Here's how the part is built. I have some questions about the finished solid (model axes, mm). A direction names the side the tool comes from. Coordinates: 2 decimals unless noted, no trailing zeros. Loops run counter-clockwise (first coordinate to the right, second up) from the corner with the lowest first, then second, coordinate; pieces in that order, holes last. Notation, with made-up numbers: (48, 23.25) -> (62, 23.25) arc R19 cw to (62, 31.25) -> close; hole circle Ø8 at (48.25, 10.5). An arc over 180 degrees is marked (long way). Answer as a JSON object with one key per item and string values. Group by question number.
Q1. I'm going to push flat-ended pins straight in: pin 1 (12 mm diameter, centred on x = 52, z = -16.5, fed in from +Y); pin 2 (2.5 mm diameter, centred on x = 1.5, z = -13.5, fed in from +Y); pin 3 (6.5 mm diameter, centred on x = 62.55, z = -35.8, fed in from +Y); pin 4 (3 mm diameter, centred on x = 62.55, z = -15, fed in from -Y). Where does each tip first touch, or does it pass through?
Q2. On a 3-axis mill with a long thin cutter (end or side, diameter ignored), from which of +Z, -Z, +X, -X, +Y, -Y can I reach the whole of each face in a straight line? I mean faces 1 (the flat face through (44, 6.35, -25)), 2 (the cylindrical face through (3.22, 29.41, -14.06)), 3 (the flat face through (3, 71, -15.175)). Say none if no direction works.
Q3. I want a section at D-D on x = 45. Write out the boundary of the cut face in (y, z).
Q4. I want a section at B-B on x = 26.35. Write out the boundary of the cut face in (y, z), then the cut area to 3 significant figures.
Q5. I need wall thicknesses on line 1 (X direction, y = 1.2, z = -15); line 2 (Z direction, x = 62.55, y = 1.2); line 3 (Y direction, x = 2.75, z = -25.4). Which ranges of each line are inside material? Lowest first, please.
Q6. Thinking about a two-plate mould opening in Z: for faces 4 (the flat face through (0, 47, -14)), 5 (the flat face through (23, 4, -50.8)), 6 (the flat face through (3, 71, -12)), 7 (the flat face through (23, 4, 0)), which applies, released by +Z, released by -Z, zero draft, split by the parting line, or undercut?
Q7. I want a section at C-C on z = -25.4. Write out the boundary of the cut face in (x, y), then the cut area to 3 significant figures.
Q8. I want a section at A-A on y = 38.1. Write out the boundary of the cut face in (x, z).
```python
from build123d import *

# Parameters (mm, degrees)
SKETCH1_W                                          = 50.8
SKETCH1_H                                          = 76.2
BOSS_EXTRUDE1_DEPTH                                = 6.35
SKETCH2_W                                          = 50.8
SKETCH2_H                                          = 6.35
BOSS_EXTRUDE2_DEPTH                                = 76.2
SKETCH3_R                                          = 14.2875
CUT_EXTRUDE1_DEPTH                                 = 7.35
CSK_FOR_10_FLAT_HEAD_SOCKET_CAP_SCREW1_D           = 5.1054
CSK_FOR_10_FLAT_HEAD_SOCKET_CAP_SCREW1_CSINK_D     = 10.4394
CSK_FOR_10_FLAT_HEAD_SOCKET_CAP_SCREW1_CSINK_ANGLE = 82
SKETCH12_W                                         = 3.175
SKETCH12_H                                         = 10.4
CUT_EXTRUDE2_DEPTH                                 = 7.35


with BuildPart() as part:
    # Sketch1 → Boss-Extrude1 (new body)
    with BuildSketch(Plane(origin=(0, 0, 0), x_dir=(0, 0, -1), z_dir=(1, 0, 0))):
        with Locations((25.4, 38.1)):
            Rectangle(SKETCH1_W, SKETCH1_H)
    extrude(amount=BOSS_EXTRUDE1_DEPTH)

    # Sketch2 → Boss-Extrude2 (add)
    with BuildSketch(Plane(origin=(6.35, 0, 0), x_dir=(0, 0, -1), z_dir=(1, 0, 0))):
        with Locations((25.4, 3.175)):
            Rectangle(SKETCH2_W, SKETCH2_H)
    extrude(amount=BOSS_EXTRUDE2_DEPTH)

    # Sketch3 → Cut-Extrude1 (cut, through all)
    with BuildSketch(Plane(origin=(6.35, 0, 0), x_dir=(0, 0, -1), z_dir=(1, 0, 0))):
        with Locations((25.4, 38.1)):
            Circle(SKETCH3_R)
    extrude(amount=-CUT_EXTRUDE1_DEPTH, mode=Mode.SUBTRACT)

    # CSK for #10 Flat Head Socket Cap Screw1 (through all)
    with Locations(Plane(origin=(0, 6.35, 0), x_dir=(1, 0, 0), z_dir=(0, 1, 0))):
        with Locations((26.35, 35.8), (62.55, 35.8), (62.55, 15), (26.35, 15)):
            CounterSinkHole(CSK_FOR_10_FLAT_HEAD_SOCKET_CAP_SCREW1_D / 2, CSK_FOR_10_FLAT_HEAD_SOCKET_CAP_SCREW1_CSINK_D / 2, counter_sink_angle=CSK_FOR_10_FLAT_HEAD_SOCKET_CAP_SCREW1_CSINK_ANGLE)

    # Sketch12 → Cut-Extrude2 (cut, through all)
    with BuildSketch(Plane(origin=(6.35, 0, 0), x_dir=(0, 0, -1), z_dir=(1, 0, 0))):
        with Locations((37.2125, 71)):
            Rectangle(SKETCH12_W, SKETCH12_H)
        with Locations((13.5875, 71)):
            Rectangle(SKETCH12_W, SKETCH12_H)
    extrude(amount=-CUT_EXTRUDE2_DEPTH, mode=Mode.SUBTRACT)


solid = part.part
```
Result set:
{
 "1": {"pin 1": "stops at y = 6.35", "pin 2": "stops at y = 65.8", "pin 3": "stops at y = 4.08", "pin 4": "passes through"},
 "2": {"face 1": "+Z, -Z, +X, +Y", "face 2": "+X, -X", "face 3": "+X, -X, +Y"},
 "3": {"outline": "(0, -50.8) -> (6.35, -50.8) -> (6.35, 0) -> (0, 0) -> close"},
 "4": {"outline": "(0, -50.8) -> (6.35, -50.8) -> (6.35, -41.02) -> (3.28, -38.35) -> (0, -38.35) -> close; (0, -33.25) -> (3.28, -33.25) -> (6.35, -30.58) -> (6.35, -20.22) -> (3.28, -17.55) -> (0, -17.55) -> close; (0, -12.45) -> (3.28, -12.45) -> (6.35, -9.78) -> (6.35, 0) -> (0, 0) -> close", "area": "241 mm²"},
 "5": {"line 1": "x = 0 to 23.8, 28.9 to 60, 65.1 to 82.55", "line 2": "z = -50.8 to -38.35, -33.25 to -17.55, -12.45 to 0", "line 3": "y = 0 to 23.81, 52.39 to 76.2"},
 "6": {"face 4": "zero draft", "face 5": "released by -Z", "face 6": "undercut", "face 7": "released by +Z"},
 "7": {"outline": "(0, 0) -> (82.55, 0) -> (82.55, 6.35) -> (6.35, 6.35) -> (6.35, 23.81) -> (0, 23.81) -> close; (0, 52.39) -> (6.35, 52.39) -> (6.35, 76.2) -> (0, 76.2) -> close", "area": "786 mm²"},
 "8": {"outline": "(0, -50.8) -> (6.35, -50.8) -> (6.35, -39.69) -> (0, -39.69) -> close; (0, -11.11) -> (6.35, -11.11) -> (6.35, 0) -> (0, 0) -> close"}
}
